Autodesk Inventor part; units mm, degrees
ref_plane "YZ Plane" through (0, 0, 0) normal (1, 0, 0) x (0, 1, 0)
ref_plane "XZ Plane" through (0, 0, 0) normal (0, 1, 0) x (-1, 0, 0)
ref_plane "XY Plane" through (0, 0, 0) normal (0, 0, 1) x (1, 0, 0)
sketch "Sketch1" plane through (0, 0, 0) normal (0, 1, 0) x (-1, 0, 0)
  line L0 (-6, 21.5) -> (6, 21.5)
  line L1 (6, 21.5) -> (6, -21.5)
  line L2 (6, -21.5) -> (-6, -21.5)
  line L3 (-6, -21.5) -> (-6, 21.5)
  line L4 (-6, 21.5) -> (6, -21.5) construction
  line L5 (6, 21.5) -> (-6, -21.5) construction
  point P0 (0, 0)
  dimension "d0" = 12
  dimension "d1" = 43
extrude "Extrusion1" add sketch "Sketch1" along normal mid plane 2.5
sketch "Sketch2" plane through (0, 1.25, 0) normal (0, 1, 0) x (1, 0, 0)
  circle A0 centre (0, -16) radius 2
  line L0 (6, 21.5) -> (-6, 21.5) construction
  line L1 (-6, 21.5) -> (-6, -21.5) construction
  line L2 (-6, -21.5) -> (6, -21.5) construction
  line L3 (6, -21.5) -> (6, 21.5) construction
  line L4 (-6, 21.5) -> (-6, -21.5) construction
  line L5 (-6, 0) -> (6, 0) construction
  circle A1 centre (0, 16) radius 2
  point P0 (0, 0)
  dimension "d4" = 4
  dimension "d5" = 16
extrude "Extrusion2" cut sketch "Sketch2" against normal through all
chamfer "Chamfer1" distance 2 angle 45 4 edges at (-6, 0, 21.5) (6, 0, 21.5) (6, 0, -21.5) (-6, 0, -21.5)
properties part number "ArmMotorSpacer"
Here's how the part is built. I have some questions about the finished solid (model axes, mm). Give positions to 0.01 mm unless a question says otherwise; leave off trailing zeros. Order: outer loops, then holes, each group sorted by start corner. A loop starts at its lowest first (then second) coordinate and runs counter-clockwise, first axis right, second up. Notation, with made-up numbers: (89.25, -4) -> (97.25, -4) arc R21 ccw to (97.25, 6) -> close; hole circle Ø5 at (46, 82.5). An arc over 180 degrees is marked (long way). One line per item, written item: value. Start each with the question number.
1. Imagine slicing it at A-A, the plane x = 0. List the corners of the cut face in (y, z) for me, plus the area to 3 significant figures.
2. Imagine slicing it at C-C, the plane z = -16. List the corners of the cut face in (x, y) for me, plus the area to 3 significant figures.
3. We'd pull the mould along Z, two halves only. Please class faces 1 (the face through (0, 0, 14)), 2 (the face through (0, 0, 21.5)), 3 (the face through (6, 0, 0)): released by +Z, released by -Z, zero draft, split by the parting line, or undercut.
4. Imagine slicing it at B-B, the plane y = -0.7. List the corners of the cut face in (x, z) for me, plus the area to 3 significant figures.
5. I need wall thicknesses on probe 1 along X at (y, z) = (0.3, 16); probe 2 along Z at (x, y) = (0, 0.2); probe 3 along Z at (x, y) = (-1.5, -1.05). Which ranges of each line are inside material? Lowest first, please. Write a range as from..to.
6. Imagine slicing it at D-D, the plane x = 5.25. List the corners of the cut face in (y, z) for me.
Values follow:
1. outline: (-1.25, -21.5) -> (1.25, -21.5) -> (1.25, -18) -> (-1.25, -18) -> close; (-1.25, -14) -> (1.25, -14) -> (1.25, 14) -> (-1.25, 14) -> close; (-1.25, 18) -> (1.25, 18) -> (1.25, 21.5) -> (-1.25, 21.5) -> close
1. area: 87.5 mm2
2. outline: (-6, -1.25) -> (-2, -1.25) -> (-2, 1.25) -> (-6, 1.25) -> close; (2, -1.25) -> (6, -1.25) -> (6, 1.25) -> (2, 1.25) -> close
2. area: 20.0 mm2
3. face 1: undercut
3. face 2: released by +Z
3. face 3: zero draft
4. outline: (-6, -19.5) -> (-4, -21.5) -> (4, -21.5) -> (6, -19.5) -> (6, 19.5) -> (4, 21.5) -> (-4, 21.5) -> (-6, 19.5) -> close; hole circle Ø4 at (0, -16); hole circle Ø4 at (0, 16)
4. area: 483 mm2
5. probe 1: x = -6..-2, 2..6
5. probe 2: z = -21.5..-18, -14..14, 18..21.5
5. probe 3: z = -21.5..-17.32, -14.68..14.68, 17.32..21.5
6. outline: (-1.25, -20.25) -> (1.25, -20.25) -> (1.25, 20.25) -> (-1.25, 20.25) -> close
